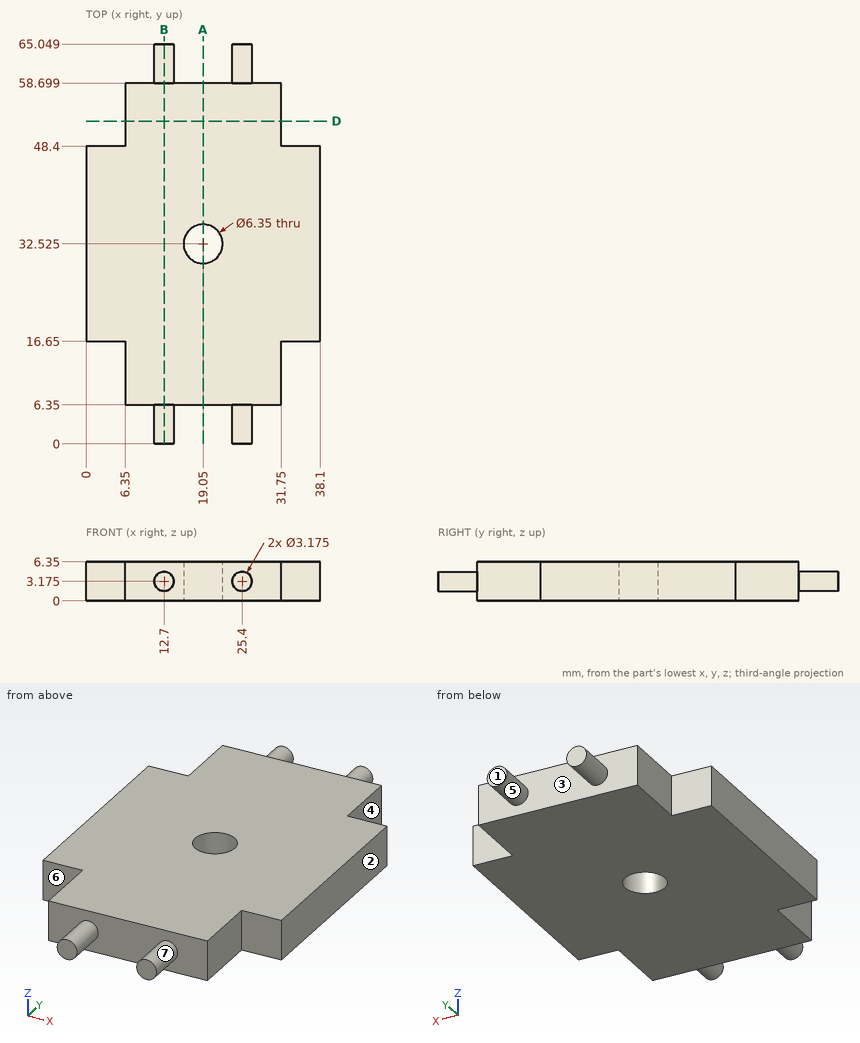
Check sheet for the drawn part. Datum: minimum x, y, z corner. Units: mm. A direction names the side the tool comes from. Round coordinates to 2 decimals unless told otherwise and drop trailing zeros. Loops run counter-clockwise (first coordinate to the right, second up) from the corner with the lowest first, then second, coordinate; pieces in that order, holes last. Notation, with made-up numbers: (13.25, -15.75) - (61.25, -15.75) arc R17 cw to (61.25, 5.25) - close; hole circle Ø11 at (-29.5, 30.5). An arc over 180 degrees is marked (long way). Write item = value, one per line. Start each with the question number.
1. Section check D-D on y = 52.5. Enter the section's corners in (x, z), then the cut area to 3 significant figures.
2. Thickness scan on line 1 (Y direction, x = 19.05, z = 5); line 2 (Y direction, x = 14, z = 1); line 3 (Y direction, x = 6, z = 5). Record the ranges inside material, lowest first.
3. Depth check by flat-ended pin: pin 1 (1.9 mm diameter, centred on x = 36.5, z = 4, fed in from -Y); pin 2 (5.5 mm diameter, centred on x = 19.05, y = 32.52, fed in from -Z); pin 3 (3 mm diameter, centred on x = 5, z = 2.5, fed in from -Y). Enter the tip coordinate at first touch or a pass-through.
4. Section check A-A on x = 19.05. Enter the section's corners in (y, z), then the cut area to 3 significant figures.
5. Section check B-B on x = 12.7. Enter the section's corners in (y, z).
6. Set-up check for the marked faces 4, 5, 6 and 7: record each of +Z, -Z, +X, -X, +Y, -Y from which the full face is reachable in a straight line by a thin tool's end or side.
7. Mould release check, pull along X, two halves, no side actions. Record for the marked faces 1, 2 and 3: released by +X, released by -X, zero draft, split by the parting line, or undercut.
Working result:
q1.outline = (6.35, 0) - (31.75, 0) - (31.75, 6.35) - (6.35, 6.35) - close
q1.area = 161 mm^2
q2.line_1 = 6.35 to 29.35, 35.7 to 58.7
q2.line_2 = 6.35 to 58.7
q2.line_3 = 16.65 to 48.4
q3.pin_1 = 16.65
q3.pin_2 = through
q3.pin_3 = 6.35
q4.outline = (6.35, 0) - (29.35, 0) - (29.35, 6.35) - (6.35, 6.35) - close; (35.7, 0) - (58.7, 0) - (58.7, 6.35) - (35.7, 6.35) - close
q4.area = 292 mm^2
q5.outline = (0, 1.59) - (6.35, 1.59) - (6.35, 0) - (58.7, 0) - (58.7, 1.59) - (65.05, 1.59) - (65.05, 4.76) - (58.7, 4.76) - (58.7, 6.35) - (6.35, 6.35) - (6.35, 4.76) - (0, 4.76) - close
q6.face_4 = +Z, -Z, +X, +Y
q6.face_5 = +Y
q6.face_6 = +Z, -Z, -X, -Y
q6.face_7 = -Y
q7.face_1 = zero draft
q7.face_2 = released by +X
q7.face_3 = undercut
